Part model, mm, in its own coordinate system. A direction names the side the tool comes from. Coordinates: 2 decimals unless noted, no trailing zeros. Write each loop counter-clockwise with the first axis right and the second up, starting at its lowest first coordinate (ties: lowest second). Pieces come first, ordered by that corner, then holes. Notation, with made-up numbers: (66, 54) -> (117, 54) arc R25 cw to (117, 92) -> close; hole circle Ø3 at (75, 45). An arc over 180 degrees is marked (long way). One line per question, with ' | ' between items. Start each with the question number.
Item 1: Two-plate mould, pull along X, no slides. Class faces 1 (the flat face through (0, 14, -39)), 2 (the flat face through (82, 15, -49)), 3 (the flat face through (30, 15, 2)): pulls with the +X half, pulls with the -X half, needs draft (parallel to the pull), parting line crosses it, or undercut.
Item 2: 3-axis set-ups, long thin cutter, end or side, ignore diameter. For faces 4 (the flat face through (76.5, 27, 0.2)), 5 (the flat face through (62, 8.3, 1.6)), 6 (the flat face through (-2, 15, -38)), 7 (the flat face through (32, 14, 0)): which of +Z, -Z, +X, -X, +Y, -Y reach the whole face in a straight line?
Item 3: Saw through at C-C (x = 43). List the corners of the cut face in (y, z).
Item 4: Saw through at D-D (z = -8.5). List the corners of the cut face in (x, y).
Item 5: Pin check, flat tips, straight feed: pin 1 (9 mm diameter, centred on x = 28.5, y = 15.5, fed in from +Z); pin 2 (5 mm diameter, centred on y = 20, z = -53, fed in from -X); pin 3 (4 mm diameter, centred on x = 52.5, y = 1.5, fed in from -Z). Stop position of each tip, or through.
Item 6: Probe probe 1 along X at (y, z) = (8, -19.5); probe 2 along Z at (x, y) = (80.5, 3); probe 3 along Z at (x, y) = (10.5, 19). List the from-to ranges inside material, lowest first. Write a range as [from, to].
Item 7: Saw through at B-B (z = -52.5). List the corners of the cut face in (x, y), and give its area (3 significant figures).
Item 8: Saw through at A-A (y = 1.5). List the corners of the cut face in (x, z), and give its area (3 significant figures).
from build123d import *

# Parameters (mm, degrees)
BOSS_EXTRUDE1_DEPTH = 30
SKETCH2_W           = 20
SKETCH2_H           = 20
CUT_EXTRUDE1_DEPTH  = 20
BOSS_EXTRUDE2_DEPTH = 2
SKETCH4_W           = 30
SKETCH4_H           = 2
CUT_EXTRUDE2_DEPTH  = 30
SKETCH5_W           = 20
SKETCH5_H           = 7
CUT_EXTRUDE3_DEPTH  = 20


with BuildPart() as part:
    # Sketch1 → Boss-Extrude1 (new body)
    with BuildSketch(Plane(origin=(0, 0, 0), x_dir=(1, 0, 0), z_dir=(0, 1, 0))):
        Polygon((0, 0), (80, 0), (80, 80), (82, 80), (82, -2), (80, -2), (-2, -2), (-2, 80), (0, 80), align=None)
    extrude(amount=BOSS_EXTRUDE1_DEPTH)

    # Sketch2 → Cut-Extrude1 (cut)
    with BuildSketch(Plane(origin=(82, 0, 0), x_dir=(0, 0, -1), z_dir=(1, 0, 0))):
        with Locations((8, 10)):
            Rectangle(SKETCH2_W, SKETCH2_H)
    extrude(amount=-CUT_EXTRUDE1_DEPTH, mode=Mode.SUBTRACT)

    # Sketch3 → Boss-Extrude2 (add)
    with BuildSketch(Plane.XZ):
        Polygon((0, -80), (-10, -80), (-10, 7.412942582), (-10, 12), (92, 12), (92, 2), (92, -80), (80, -80), (80, 0), (0, 0), align=None)
    extrude(amount=BOSS_EXTRUDE2_DEPTH)

    # Sketch4 → Cut-Extrude2 (cut)
    with BuildSketch(Plane(origin=(92, 0, 0), x_dir=(0, 0, -1), z_dir=(1, 0, 0))):
        with Locations((3, -1)):
            Rectangle(SKETCH4_W, SKETCH4_H)
    extrude(amount=-CUT_EXTRUDE2_DEPTH, mode=Mode.SUBTRACT)

    # Sketch5 → Cut-Extrude3 (cut)
    with BuildSketch(Plane(origin=(82, 0, 0), x_dir=(0, 0, -1), z_dir=(1, 0, 0))):
        with Locations((8, 23.5)):
            Rectangle(SKETCH5_W, SKETCH5_H)
    extrude(amount=-CUT_EXTRUDE3_DEPTH, mode=Mode.SUBTRACT)


solid = part.part
From the geometry:
1) face 1: undercut | face 2: pulls with the +X half | face 3: needs draft
2) face 4: +Z, +X, -Y | face 5: +Z, -Z, +X, -Y | face 6: +Z, -Z, -X, +Y | face 7: -Z, +Y, -Y
3) outline: (-2, 0) -> (30, 0) -> (30, 2) -> (0, 2) -> (0, 12) -> (-2, 12) -> close
4) outline: (-10, -2) -> (0, -2) -> (0, 30) -> (-2, 30) -> (-2, 0) -> (-10, 0) -> close; (80, 27) -> (82, 27) -> (82, 30) -> (80, 30) -> close
5) pin 1: z = 2 | pin 2: x = -2 | pin 3: z = 0
6) probe 1: [-2, 0], [80, 82] | probe 2: [-80, -18] | probe 3: [0, 2]
7) outline: (-10, -2) -> (0, -2) -> (0, 30) -> (-2, 30) -> (-2, 0) -> (-10, 0) -> close; (80, -2) -> (92, -2) -> (92, 0) -> (82, 0) -> (82, 30) -> (80, 30) -> close | area: 164 mm2
8) outline: (-2, -80) -> (0, -80) -> (0, 0) -> (62, 0) -> (62, 2) -> (-2, 2) -> close; (80, -80) -> (82, -80) -> (82, -18) -> (80, -18) -> close | area: 412 mm2
